Source: CAD feature listing. Evaluate the final solid. Frame: model axes, mm. A direction names the side the tool comes from. Give positions to 0.01 mm unless a question says otherwise; leave off trailing zeros. Loops run counter-clockwise (first coordinate to the right, second up) from the corner with the lowest first, then second, coordinate; pieces in that order, holes last. Notation, with made-up numbers: M 71.5,-9 L 125.5,-9 A26 cw 125.5,30 Z; hole C -3,-12 d1. An arc over 180 degrees is marked long. Write item = value, one per line.
Autodesk Inventor part; units mm, degrees
ref_plane "Work Plane1" through (-24.9, -24.9, 7.7) normal (0, 0, 1) x (1, 0, 0)
ref_plane "Work Plane2" through (24.825, 0, 41.65) normal (0.9848078, 0, -0.1736482) x (0, 1, 0)
ref_plane "YZ Plane" through (0, 0, 0) normal (1, 0, 0) x (0, 1, 0)
ref_plane "Work Plane1" through (-24.9, -24.9, 7.7) normal (0, 0, 1) x (1, 0, 0)
sketch "Sketch1" plane through (0, 0, 0) normal (0, 0, 1) x (0, 1, 0)
  circle A0 centre (20.9, 10) radius 1.875
  circle A1 centre (-20.9, 10) radius 1.875
  circle A2 centre (20.9, -10) radius 1.875
  circle A3 centre (-20.9, -10) radius 1.875
  circle A4 centre (-14.4, -20.8) radius 2.0675
  circle A5 centre (14.4, -20.8) radius 2.0675
  circle A6 centre (14.4, 20.8) radius 2.0675
  circle A7 centre (-14.4, 20.8) radius 2.0675
  line L0 (-16.9, -16.9) -> (-16.9, 16.9)
  line L1 (-16.9, 16.9) -> (16.9, 16.9)
  line L2 (16.9, 16.9) -> (16.9, -16.9)
  line L3 (16.9, -16.9) -> (-16.9, -16.9)
  line L4 (24.9, 17.05) -> (22.55, 17.05)
  line L5 (22.55, 17.05) -> (17.05, 22.55)
  line L6 (17.05, 22.55) -> (17.05, 24.9)
  line L7 (17.05, 24.9) -> (-17.05, 24.9)
  line L8 (-17.05, 24.9) -> (-17.05, 22.55)
  line L9 (-17.05, 22.55) -> (-22.55, 17.05)
  line L10 (-22.55, 17.05) -> (-24.9, 17.05)
  line L11 (-24.9, 17.05) -> (-24.9, -17.05)
  line L12 (-24.9, -17.05) -> (-22.55, -17.05)
  line L13 (-22.55, -17.05) -> (-17.05, -22.55)
  line L14 (-17.05, -22.55) -> (-17.05, -24.9)
  line L15 (-17.05, -24.9) -> (17.05, -24.9)
  line L16 (17.05, -24.9) -> (17.05, -22.55)
  line L17 (17.05, -22.55) -> (22.55, -17.05)
  line L18 (22.55, -17.05) -> (24.9, -17.05)
  line L19 (24.9, -17.05) -> (24.9, 17.05)
  line L20 (16.975, -24.825) -> (-16.975, -24.825)
  line L21 (-16.975, -24.825) -> (-16.975, -22.5189)
  line L22 (-16.975, -22.5189) -> (-22.5189, -16.975)
  line L23 (-22.5189, -16.975) -> (-24.825, -16.975)
  line L24 (-24.825, -16.975) -> (-24.825, 16.975)
  line L25 (-24.825, 16.975) -> (-22.5189, 16.975)
  line L26 (-22.5189, 16.975) -> (-16.975, 22.5189)
  line L27 (-16.975, 22.5189) -> (-16.975, 24.825)
  line L28 (-16.975, 24.825) -> (16.975, 24.825)
  line L29 (16.975, 24.825) -> (16.975, 22.5189)
  line L30 (16.975, 22.5189) -> (22.5189, 16.975)
  line L31 (22.5189, 16.975) -> (24.825, 16.975)
  line L32 (24.825, 16.975) -> (24.825, -16.975)
  line L33 (24.825, -16.975) -> (22.5189, -16.975)
  line L34 (22.5189, -16.975) -> (16.975, -22.5189)
  line L35 (16.975, -22.5189) -> (16.975, -24.825)
  dimension "d5" = 0.075
extrude "Extrusion1" add sketch "Sketch1" along normal blind 2.5 from surface at 7.7 contours A0 | A1 | A2 | A3 | A4 | A5 | A6 | A7 | L0 L1 L2 L3 | L20 L21 L22 L23 L24 L25 L26 L27 L28 L29 L30 L31 L32 L33 L34 L35
sketch "Sketch2" plane through (0, 0, 0) normal (0, 1, 0) x (-1, 0, 0)
  line L0 (16.975, 10.2) -> (-16.975, 10.2)
  line L1 (-16.975, 7.7) -> (-16.975, 10.2)
  line L2 (16.975, 7.7) -> (-16.975, 7.7)
  line L3 (16.975, 7.7) -> (16.975, 10.2)
  line L4 (16.975, 7.7) -> (-16.975, 41.65)
  line L5 (16.975, 7.7) -> (64.9876, 7.7) construction
  line L6 (-16.975, 41.65) -> (-16.975, 10.2)
  line L7 (-20.5105, 41.65) -> (10.9395, 10.2)
  line L8 (7.4039, 10.2) -> (-24.0461, 41.65)
  line L9 (-19.475, 12.7) -> (19.475, 12.7)
  line L10 (19.475, 12.7) -> (19.475, 5.2)
  line L11 (19.475, 5.2) -> (-19.475, 5.2)
  line L12 (-19.475, 5.2) -> (-19.475, 12.7)
  line L13 (-16.975, 41.65) -> (-24.825, 41.65)
  line L14 (-24.825, 41.65) -> (-24.825, 10.2)
  line L15 (-24.825, 10.2) -> (-16.975, 10.2)
  line L16 (-16.975, 10.2) -> (-16.975, 41.65)
  point P0 (0, 0)
  point P1 (14.475, 10.2)
  point P2 (-16.975, 38.1145)
  point P3 (-16.975, 34.5789)
  point P4 (8.4395, 12.7)
  point P5 (11.975, 12.7)
  point P6 (-19.475, 10.2)
  point P7 (-16.975, 12.7)
  point P8 (-16.975, 10.2)
  dimension "d6" = 135
  dimension "d9" = 2.5
  dimension "d10" = 2.5
  dimension "d13" = 2.5
extrude "Extrusion2" add sketch "Sketch2" along normal mid plane 30 contours L7 L9 L4 L0 | L0 L8 L9 L7 | L0 L6 L9 L8 | L9 L8 L6 L7 | L7 L6 L4 L9 | L15 L12 L9 L6 | L9 L6 L8 | L7 L13 L6 | L6 L8 L13 L7 | L9 L12 L15 L14 L13 L8 L6
extrude "Extrusion3" cut sketch "Sketch2" along normal mid plane 30 contours L7 L9 L4 L0 | L0 L8 L9 L7 | L9 L8 L6 L7 | L7 L13 L6 | L6 L8 L13 L7
ref_plane "Work Plane2" through (24.825, 0, 41.65) normal (0.9848078, 0, -0.1736482) x (0, 1, 0)
sketch "Sketch3" plane through (20.7643, -15, 18.6207) normal (0.9848078, 0, -0.1736482) x (-0.1736482, 0, -0.9848078)
  line L0 (10.902, 0) -> (-18.5396, 0)
  line L1 (10.902, 0) -> (10.902, 30)
  line L2 (-18.5396, 30) -> (10.902, 30)
  line L3 (-18.5396, 15) -> (10.902, 15)
  line L4 (6.1812, 6.25) -> (-13.8188, 6.25)
  line L5 (-13.8188, 6.25) -> (-13.8188, 23.75)
  line L6 (-13.8188, 23.75) -> (6.1812, 23.75)
  line L7 (6.1812, 23.75) -> (6.1812, 6.25)
  line L8 (6.1812, 6.25) -> (-13.8188, 23.75) construction
  line L9 (-13.8188, 6.25) -> (6.1812, 23.75) construction
  circle A0 centre (-13.8188, 6.25) radius 2.5875
  circle A1 centre (-13.8188, 6.25) radius 5.0875
  line L10 (-3.8188, 15) -> (-3.8188, 6.25)
  line L11 (-3.8188, 10.625) -> (-13.8188, 10.625)
  line L12 (-8.8188, 10.625) -> (-8.8188, 6.25)
  circle A2 centre (-13.8188, 15) radius 2.5875
  circle A3 centre (-13.8188, 15) radius 5.0875
  circle A4 centre (-3.8188, 15) radius 5.0875
  circle A5 centre (-3.8188, 15) radius 2.5875
  line L13 (-18.9063, 6.25) -> (-18.9063, 15)
  line L14 (-8.7313, 15) -> (-8.7313, 6.25)
  line L15 (-18.5396, 0) -> (-18.5396, 30)
  point P0 (21.9435, 15)
  dimension "d16" = 20
  dimension "d17" = 17.5
  dimension "d18" = 5.175
  dimension "d19" = 2.5
extrude "Extrusion4" cut sketch "Sketch3" along normal mid plane 50 contours A0 L5 L4 | L4 L5 A0 | A2 L3 L5 | L5 L3 A2 | A2 L5 L3 | A2 L3 L5
extrude "Extrusion5" cut sketch "Sketch3" along normal blind 4.25 and the other way blind 2.5 contours L15 A1 A3 L5 A0 L4 | A1 L15 | L13 A3 L15 A1 | L4 L12 A1 | A1 L12 L11 L14 | L15 A3 A1 | A3 L15 | L4 A0 L5 A3 A1 L12 | A1 L11 L12 | L11 A3 A4 L14 | A3 L15 L3 A2 L5 A1 | A1 L5 A3 | A3 L5 A2 L3 L15 | A4 L3 A2 L5 A3 | A3 L3 A4 | A0 L5 L4 | L4 L5 A0 | L11 L5 A1 | A3 L5 L11 | A1 L5 A2 L3 A4 A3 | A4 A3 L14 | A3 A4 L3 | A2 L3 L5 | L5 L3 A2 | A2 L5 L3 | A2 L3 L5
sketch "Sketch4" plane through (17.8921, 0, 2.3313) normal (0.9848078, 0, -0.1736482) x (0, 1, 0)
  line L0 (-15, 5.6387) -> (-15, 35.0803)
  line L1 (-15, 5.6387) -> (15, 5.6387)
  line L2 (15, 35.0803) -> (15, 5.6387)
  circle A0 centre (0, 14.3887) radius 2.5875
  circle A1 centre (0, 14.3887) radius 5.0875
  line L3 (-15, 35.0803) -> (15, 35.0803)
  line L4 (0, 5.6387) -> (0, 14.3887)
  point P0 (0, -5.1645)
  dimension "d25" = 5.175
  dimension "d26" = 2.5
  dimension "d37" = 8.75
extrude "Extrusion6" cut sketch "Sketch4" along normal mid plane 100 contours A0
extrude "Extrusion7" cut sketch "Sketch4" along normal blind 15 and the other way blind 10 contours A0 | A1
sketch "Sketch7" plane through (-3.5875, 0, 17.552) normal (0, 1, 0) x (-0.7071068, 0, -0.7071068)
  line L0 (-20.158, 0) -> (-26.4755, 0)
  line L1 (-0.6613, 0) -> (-6.9788, 0)
  line L2 (1.0892, 2.5) -> (-0.6613, 0)
  line L3 (-5.2283, 2.5) -> (1.0892, 2.5)
  line L4 (-5.2283, 2.5) -> (-6.9788, 0)
  line L5 (-18.4075, 2.5) -> (-20.158, 0)
  line L6 (-24.725, 2.5) -> (-18.4075, 2.5)
  line L7 (-24.725, 2.5) -> (-26.4755, 0)
  line L8 (-3.8201, 0) -> (-4.0701, 0)
  line L9 (-23.3168, 0) -> (-23.5668, 0)
  line L10 (-1.7448, -1.4254) -> (-6.7427, -0.5442)
  line L11 (-6.7427, -0.5442) -> (-6.3954, 1.4254)
  line L12 (-6.3954, 1.4254) -> (-1.3975, 0.5442)
  line L13 (-1.3975, 0.5442) -> (-1.7448, -1.4254)
  line L14 (-1.7448, -1.4254) -> (-6.3954, 1.4254) construction
  line L15 (-6.7427, -0.5442) -> (-1.3975, 0.5442) construction
  line L16 (-1.7448, -1.4254) -> (3.3302, -1.4254) construction
  line L17 (-21.2415, -1.4254) -> (-26.2394, -0.5442)
  line L18 (-26.2394, -0.5442) -> (-25.8921, 1.4254)
  line L19 (-25.8921, 1.4254) -> (-20.8942, 0.5442)
  line L20 (-20.8942, 0.5442) -> (-21.2415, -1.4254)
  line L21 (-21.2415, -1.4254) -> (-25.8921, 1.4254) construction
  line L22 (-26.2394, -0.5442) -> (-20.8942, 0.5442) construction
  line L23 (-21.2415, -1.4254) -> (-16.1665, -1.4254) construction
  line L24 (-27.1088, 3.1631) -> (-27.9771, -1.7609)
  line L25 (-27.9771, -1.7609) -> (-20.0247, -3.1631)
  line L26 (-20.0247, -3.1631) -> (-19.1565, 1.7609)
  line L27 (-19.1565, 1.7609) -> (-27.1088, 3.1631)
  line L28 (-7.6121, 3.1631) -> (-8.4804, -1.7609)
  line L29 (-8.4804, -1.7609) -> (-0.528, -3.1631)
  line L30 (-0.528, -3.1631) -> (0.3402, 1.7609)
  line L31 (0.3402, 1.7609) -> (-7.6121, 3.1631)
  line L32 (-0.6613, 0) -> (0.0297, 0)
  line L33 (-20.158, 0) -> (-19.467, 0)
  line L34 (-1.7448, -1.4254) -> (0.0297, 0)
  line L35 (-21.2415, -1.4254) -> (-19.467, 0)
  line L36 (-26.4755, 0) -> (-27.6666, 0)
  line L37 (-6.9788, 0) -> (-8.1699, 0)
  line L38 (-6.7427, -0.5442) -> (-8.1699, 0)
  line L39 (-26.2394, -0.5442) -> (-27.6666, 0)
  point P0 (-1.4934, 0)
  point P1 (-6.6467, 0)
  point P2 (-26.1434, 0)
  point P3 (-20.9901, 0)
  dimension "d70" = 0.25
  dimension "d71" = 0.25
  dimension "d72" = 5.075
  dimension "d73" = 170
  dimension "d74" = 2
  dimension "d75" = 5.075
  dimension "d76" = 170
  dimension "d77" = 2
  dimension "d78" = 1.5
  dimension "d79" = 1.5
extrude "Extrusion10" add sketch "Sketch7" along normal mid plane 30 contours L0 L18 L7 L19 L20 | L20 L19 L7 L6 L27 L26 L5 L0 | L0 L7 L18 | L26 L27 L6 L5 | L1 L11 L4 L12 L13 | L13 L12 L4 L3 L31 L30 L2 L1 | L1 L4 L11 | L30 L31 L3 L2
extrude "Extrusion11" cut sketch "Sketch7" along normal mid plane 5.075 contours L0 L20 L17 L18 | L0 L18 L7 L19 L20 | L18 L19 L7 | L1 L13 L10 L11 | L1 L11 L4 L12 L13 | L11 L12 L4
sketch "Sketch8" plane through (13.713, -15.0375, 36.8684) normal (0.819152, 0, -0.5735764) x (-0.5735764, 0, -0.819152)
  line L0 (0, 12.5) -> (0, 17.575)
  line L1 (5.075, 17.575) -> (5.075, 12.5)
  line L2 (0, 12.5) -> (5.075, 12.5)
  line L3 (5.075, 17.575) -> (0, 17.575)
  line L4 (2.5375, 12.5) -> (2.5375, 17.575)
  circle A0 centre (2.5375, 15.0375) radius 2.5375
  circle A1 centre (2.5375, 15.0375) radius 4.0375
  circle A2 centre (2.5375, 6.2875) radius 4.0375
  circle A3 centre (2.5375, 6.2875) radius 2.5375
  line L5 (-1.5, 6.2875) -> (-1.5, 15.0375)
  line L6 (6.575, 6.2875) -> (6.575, 15.0375)
  point P0 (38.0663, 15.0375)
  dimension "d86" = 5.075
  dimension "d87" = 1.5
  dimension "d90" = 8.75
extrude "Extrusion12" cut sketch "Sketch8" along normal blind 1.5 contours A0 L4 | L4 A0 | A3
extrude "Extrusion13" add sketch "Sketch8" along normal blind 1.5 contours L0 A0 L2 | L0 L3 A0 | A0 L1 L2 | L3 L1 A0 | A1 | L6 A2 L5 A1 | A2
sketch "Sketch9" plane through (-0.0732, -2.5375, 23.0821) normal (0.819152, 0, -0.5735764) x (-0.5735764, 0, -0.819152)
  line L0 (0, 0) -> (0, 5.075)
  line L1 (0, 0) -> (5.075, 0)
  line L2 (5.075, 5.075) -> (5.075, 0)
  line L3 (5.075, 5.075) -> (0, 5.075)
  line L4 (2.5375, 0) -> (2.5375, 5.075)
  circle A0 centre (2.5375, 2.5375) radius 2.5375
  circle A1 centre (2.5375, 2.5375) radius 4.0375
  point P0 (18.8658, 2.5375)
  dimension "d99" = 5.075
  dimension "d100" = 1.5
extrude "Extrusion14" add sketch "Sketch9" along normal blind 1.5 contours L0 A0 L1 | L0 L3 A0 | A0 L2 L1 | L3 L2 A0 | A1
chamfer "Chamfer1" distance 1.21 angle 45 3 edges at (11.9583, -12.4749, 33.0978) (-1.8279, 3.7249, 19.3115) (-1.8279, -3.7249, 19.3115)
sketch "Sketch10" plane through (0, 0, 0) normal (0, 1, 0) x (-1, 0, 0)
  line L0 (8.4395, 12.7) -> (-16.975, 38.1145)
  line L1 (-16.975, 38.1145) -> (-16.975, 41.65)
  line L2 (-16.975, 41.65) -> (11.975, 12.7)
  line L3 (11.975, 12.7) -> (8.4395, 12.7)
  line L4 (-11.1764, 30.6305) -> (-15.1128, 36.2522)
  line L5 (-11.1689, 30.6232) -> (-11.1764, 30.6305)
  line L6 (-15.1128, 36.2522) -> (-9.3221, 30.4616)
  line L7 (-1.3265, 22.466) -> (2.6099, 16.8443)
  line L8 (2.6099, 16.8443) -> (2.6099, 16.8443)
  line L9 (2.6099, 16.8443) -> (-1.3265, 22.466)
  line L10 (-1.3265, 22.466) -> (-1.3265, 22.466)
  line L11 (-24.0461, 41.65) -> (7.4039, 10.2)
  line L12 (-24.825, 10.2) -> (7.4039, 10.2)
  line L13 (-24.825, 10.2) -> (-24.825, 41.65)
  line L14 (-24.825, 41.65) -> (-24.0461, 41.65)
  line L15 (22.5189, 10.2) -> (24.825, 10.2)
  line L16 (24.825, 7.7) -> (24.825, 10.2)
  line L17 (22.5189, 7.7) -> (24.825, 7.7)
  line L18 (22.5189, 7.7) -> (22.5189, 10.2)
  line L19 (16.975, 10.2) -> (22.5189, 10.2)
  line L20 (22.5189, 7.7) -> (22.5189, 10.2)
  line L21 (16.975, 7.7) -> (22.5189, 7.7)
  line L22 (16.975, 7.7) -> (16.975, 10.2)
  line L23 (-16.975, 10.2) -> (16.975, 10.2)
  line L24 (16.975, 7.7) -> (16.975, 10.2)
  line L25 (-16.975, 7.7) -> (16.975, 7.7)
  line L26 (-16.975, 7.7) -> (-16.975, 10.2)
  line L27 (-22.5189, 10.2) -> (-16.975, 10.2)
  line L28 (-16.975, 7.7) -> (-16.975, 10.2)
  line L29 (-22.5189, 7.7) -> (-16.975, 7.7)
  line L30 (-22.5189, 7.7) -> (-22.5189, 10.2)
  line L31 (-24.825, 10.2) -> (-22.5189, 10.2)
  line L32 (-22.5189, 7.7) -> (-22.5189, 10.2)
  line L33 (-24.825, 7.7) -> (-22.5189, 7.7)
  line L34 (-24.825, 7.7) -> (-24.825, 10.2)
  line L35 (2.6099, 16.8443) -> (8.4395, 12.7)
  line L36 (-11.1764, 30.6305) -> (-1.3265, 22.466)
  line L37 (-11.1689, 30.6232) -> (-9.3221, 30.4616)
  point P0 (0, 0)
extrude "Extrusion15" cut sketch "Sketch10" along normal mid plane 50 contours L11 L12 L13 L14 | L23 L22 L25 L26 L12 | L26 L29 L30 L12 | L19 L18 L21 L22 | L12 L30 L33 L34 | L15 L16 L17 L18
properties part number "Mirror Plate"
1. Cut plane B-B, the plane z = 23.75. Return the cut outline in (x, y) (1 decimal).
Derived:
outline = M -0.9,-15 L 2.6,-15 L 2.6,15 L -0.9,15 Z
2. Cut plane C-C, the plane x = -7.25. Return the cut outline in (y, z) (1 decimal), then the cut area to 3 significant figures.
Derived:
outline = M -15,13.9 L 15,13.9 L 15,17.4 L -15,17.4 Z
area = 106 mm²
3. Pull-direction query (Y, two-part tool) for faces 1 (the flat face through (4.45, -0.21, 25.59)), 2 (the flat face through (4, 15, 26)), 3 (the cylindrical face through (12.2, -6.5, 33.4)), 4 (the cylindrical face through (0.531, -0.112, 22.656)); classes: +Y half, -Y half, draft (parallel to the pull), parting line (faces both ways), or undercut.
Derived:
face_1 = draft
face_2 = +Y half
face_3 = undercut
face_4 = undercut
4. First-contact query: pin 1 Ø4 at (y, z) = (-5, 35) entering from -X (3 decimals); pin 2 Ø10 at (x, y) = (2, 2) entering from +Z (3 decimals); pin 3 Ø1 at (x, y) = (7.5, 4.5) entering from -Z. Flat tips, straight axial feed; report the tip coordinate or a pass-through.
Derived:
pin_1 = 8.325
pin_2 = 31.675
pin_3 = 28.14
5. Material intervals for probe 1 along X at (y, z) = (-4, 24.5) (1 decimal); probe 2 along Z at (x, y) = (-1.25, -8.5) (1 decimal); probe 3 along X at (y, z) = (-6.5, 32.5) (3 decimals), sorted ascending. Write a range as from..to.
Derived:
probe_1 = -0.2..3.4
probe_2 = 19.9..23.4
probe_3 = 7.825..12.485
6. Reachability of faces 5 (the flat face through (4, -15, 26)), 6 (the flat face through (-1.51, -0.04, 21.03)) from +Z, -Z, +X, -X, +Y, -Y: full face, straight path, thin tool, end or side. Return the list, or none.
Derived:
face_5 = +Z, -Z, +X, -X, -Y
face_6 = none
